```python
from build123d import *

# Parameters (mm, degrees)
F0_W     = 914.4
F0_H     = 304.8
F0_W_2   = 38.1
F0_H_2   = 152.4
F0_W_3   = 8.255
F1_DEPTH = 17.526
F2_DEPTH = 6.35


with BuildPart() as f1:
    # F0 (on Top) → F1 (new body)
    with BuildSketch(Plane.XY):
        with Locations((0, -1.919626)):
            Rectangle(F0_W, F0_H)
        with Locations((-387.35, 0)):
            Rectangle(F0_W_2, F0_H_2, mode=Mode.SUBTRACT)
        with Locations((-247.65, 0)):
            Rectangle(F0_W_2, F0_H_2, mode=Mode.SUBTRACT)
        with Locations((247.65, 0)):
            Rectangle(F0_W_2, F0_H_2, mode=Mode.SUBTRACT)
        with Locations((387.35, 0)):
            Rectangle(F0_W_2, F0_H_2, mode=Mode.SUBTRACT)
        with Locations((-461.3275, -1.919626)):
            Rectangle(F0_W_3, F0_H)
        with Locations((461.3275, -1.919626)):
            Rectangle(F0_W_3, F0_H)
    extrude(amount=F1_DEPTH)

    # F0 (on Top) → F2 (join)
    with BuildSketch(Plane.XY):
        with Locations((-387.35, 0)):
            Rectangle(F0_W_2, F0_H_2)
        with Locations((-247.65, 0)):
            Rectangle(F0_W_2, F0_H_2)
        with Locations((247.65, 0)):
            Rectangle(F0_W_2, F0_H_2)
        with Locations((387.35, 0)):
            Rectangle(F0_W_2, F0_H_2)
    extrude(amount=F2_DEPTH)


solid = f1.part
```
Here's how the part is built. I have some questions about the finished solid (model axes, mm). A direction names the side the tool comes from. Coordinates: 2 decimals unless noted, no trailing zeros. Order: outer loops, then holes, each group sorted by start corner. A loop starts at its lowest first (then second) coordinate and runs counter-clockwise, first axis right, second up.
Item 1: I'm going to push a flat-ended pin straight in: pin 1 Ø19 at (x, y) = (386.5, 22.5) entering from +Z. Where does the tip first touch, or does it pass through?
Response values:
pin 1: stops at z = 6.35
Item 2: Which directions (+Z, -Z, +X, -X, +Y, -Y) give clear straight access to the entire face, cutting with the end or side of a thin tool? Please do faces 4 (the face through (-248, 1, 6.35)), 5 (the face through (-7, 0, 0)).
Response values:
face 4: +Z
face 5: -Z, +X, -X, +Y, -Y
Item 3: If we section it at B-B, the plane z = 9.5: List the corners of the cut face in (x, y) for me (3 decimals).
Response values:
outline: (-465.455, -154.32) - (465.455, -154.32) - (465.455, 150.48) - (-465.455, 150.48) - close; hole (-406.4, -76.2) - (-368.3, -76.2) - (-368.3, 76.2) - (-406.4, 76.2) - close; hole (-266.7, -76.2) - (-228.6, -76.2) - (-228.6, 76.2) - (-266.7, 76.2) - close; hole (228.6, -76.2) - (266.7, -76.2) - (266.7, 76.2) - (228.6, 76.2) - close; hole (368.3, -76.2) - (406.4, -76.2) - (406.4, 76.2) - (368.3, 76.2) - close
Item 4: Thinking about a two-plate mould opening in X: for faces 1 (the face through (-388, 1, 6.35)), 2 (the face through (465.455, -4, 9)), 3 (the face through (7, 150.48, 9)), which applies, pulls with the +X half, pulls with the -X half, needs draft (parallel to the pull), parting line crosses it, or undercut?
Response values:
face 1: undercut
face 2: pulls with the +X half
face 3: needs draft
Item 5: I need wall thicknesses on probe 1 along X at (y, z) = (11.5, 12.25) (3 decimals); probe 2 along Y at (x, z) = (379, 11.75); probe 3 along Z at (x, y) = (230.5, -1). Which ranges of each line are inside material? Lowest first, please.
Response values:
probe 1: x = -465.455 to -406.4, -368.3 to -266.7, -228.6 to 228.6, 266.7 to 368.3, 406.4 to 465.455
probe 2: y = -154.32 to -76.2, 76.2 to 150.48
probe 3: z = 0 to 6.35
Item 6: If we section it at A-A, the plane y = -50: List the corners of the cut face in (x, z) for me (3 decimals).
Response values:
outline: (-465.455, 0) - (465.455, 0) - (465.455, 17.526) - (406.4, 17.526) - (406.4, 6.35) - (368.3, 6.35) - (368.3, 17.526) - (266.7, 17.526) - (266.7, 6.35) - (228.6, 6.35) - (228.6, 17.526) - (-228.6, 17.526) - (-228.6, 6.35) - (-266.7, 6.35) - (-266.7, 17.526) - (-368.3, 17.526) - (-368.3, 6.35) - (-406.4, 6.35) - (-406.4, 17.526) - (-465.455, 17.526) - close
Item 7: If we section it at C-C, the plane x = -252: List the corners of the cut face in (y, z) for me, then the cut area to 3 significant figures.
Response values:
outline: (-154.32, 0) - (150.48, 0) - (150.48, 17.53) - (76.2, 17.53) - (76.2, 6.35) - (-76.2, 6.35) - (-76.2, 17.53) - (-154.32, 17.53) - close
area: 3,640 mm2
